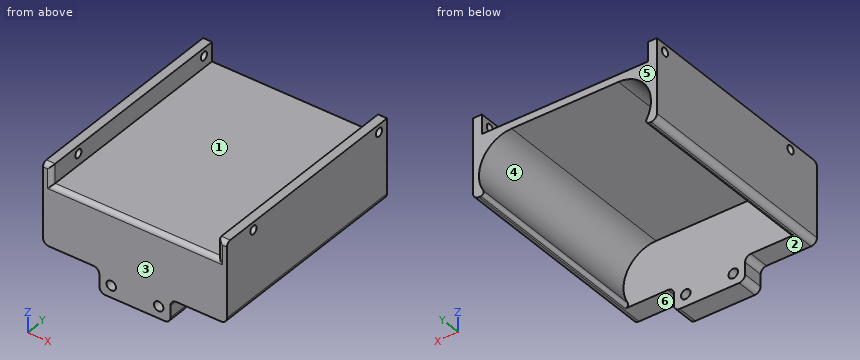
```python
from build123d import *

# Parameters (mm, degrees)
BOSS_EXTRUDE1_DEPTH = 72
CUT_EXTRUDE1_DEPTH  = 65
FILLET3_R           = 2
FILLET4_R           = 1.5
SKETCH5_R           = 1.4
CUT_EXTRUDE2_DEPTH  = 96.970047411
SKETCH6_W           = 24
SKETCH6_H           = 8
BOSS_EXTRUDE3_DEPTH = 7
FILLET5_R           = 2
SKETCH7_R           = 1.6
CUT_EXTRUDE3_DEPTH  = 7
FILLET6_R           = 1


with BuildPart() as part:
    # Sketch1 → Boss-Extrude1 (new body)
    with BuildSketch(Plane(origin=(0, 0, 0), x_dir=(1, 0, 0), z_dir=(0, 1, 0))):
        Polygon((-31, 13.5), (-31, -13.5), (-28, -13.5), (-28, -7), (28, -7), (28, -13.5), (31, -13.5), (31, 13.5), (28, 13.5), (-28, 13.5), align=None)
    extrude(amount=BOSS_EXTRUDE1_DEPTH)

    # Sketch2 → Cut-Extrude1 (cut)
    with BuildSketch(Plane(origin=(0, 72, 0), x_dir=(1, 0, 0), z_dir=(0, 1, 0))):
        with BuildLine():
            Line((17.999983181, 17.5), (-18.000016819, 17.500086496))
            ThreePointArc((-18.000016819, 17.500086496), (-29.000086496, 6.499978376), (-17.999973571, -4.500086496))
            Line((-17.999973571, -4.500086496), (18.000026429, -4.5))
            ThreePointArc((18.000026429, -4.5), (29, 6.500021624), (17.999983181, 17.5))
        make_face()
    extrude(amount=-CUT_EXTRUDE1_DEPTH, mode=Mode.SUBTRACT)

    # Fillet3
    fillet3_edges = [part.edges().sort_by_distance(p)[0] for p in [
        (31, 36, -13.5),
        (-31, 36, -13.5),
    ]]
    fillet(fillet3_edges, radius=FILLET3_R)

    # Fillet4
    fillet4_edges = [part.edges().sort_by_distance(p)[0] for p in [
        (29.5, 0, 13.5),
        (28, 0, 10.25),
        (0, 0, 7),
        (-28, 0, 10.25),
        (-29.5, 0, 13.5),
    ]]
    fillet(fillet4_edges, radius=FILLET4_R)

    # Sketch5 → Cut-Extrude2 (cut, through all)
    with BuildSketch(Plane.ZY.offset(31)):
        with Locations((10.9, 68.4)):
            Circle(SKETCH5_R)
        with Locations((10.9, 11.9)):
            Circle(SKETCH5_R)
    extrude(amount=-CUT_EXTRUDE2_DEPTH, mode=Mode.SUBTRACT)

    # Sketch6 → Boss-Extrude3 (add)
    with BuildSketch(Plane(origin=(0, 0, 0), x_dir=(1, 0, 0), z_dir=(0, 1, 0))):
        with Locations((-5.6065e-05, 17.5)):
            Rectangle(SKETCH6_W, SKETCH6_H)
    extrude(amount=BOSS_EXTRUDE3_DEPTH)

    # Fillet5
    fillet5_edges = [part.edges().sort_by_distance(p)[0] for p in [
        (-12.000056065, 3.5, -21.5),
        (-12.000056065, 3.5, -13.5),
        (11.999943935, 3.5, -13.5),
        (11.999943935, 3.5, -21.5),
    ]]
    fillet(fillet5_edges, radius=FILLET5_R)

    # Sketch7 → Cut-Extrude3 (cut)
    with BuildSketch(Plane(origin=(0, 7, 0), x_dir=(1, 0, 0), z_dir=(0, 1, 0))):
        with Locations(Location((-8.000056065, 17.5, 0), (0, 0, 270))):
            Circle(SKETCH7_R)
        with Locations(Location((7.999943935, 17.5, 0), (0, 0, 270))):
            Circle(SKETCH7_R)
    extrude(amount=-CUT_EXTRUDE3_DEPTH, mode=Mode.SUBTRACT)

    # Fillet6
    fillet6_edges = [part.edges().sort_by_distance(p)[0] for p in [
        (26.485281374, 39.5, -13.5),
        (-26.485393504, 39.5, -13.5),
    ]]
    fillet(fillet6_edges, radius=FILLET6_R)


solid = part.part
```
Model file for the job. Use its own axes, mm. Face numbers are marked on the shaded views. A direction names the side the tool comes from. Round coordinates to 2 decimals unless told otherwise and drop trailing zeros. Write each loop counter-clockwise with the first axis right and the second up, starting at its lowest first coordinate (ties: lowest second). Pieces come first, ordered by that corner, then holes. Notation, with made-up numbers: (-33.75, -18.5) - (-6.75, -18.5) arc R17 ccw to (-6.75, -4.5) - close; hole circle Ø9 at (66, 42.5). An arc over 180 degrees is marked (long way). One line per item, written item: value.
(1) Wall check: probe 1 along X at (y, z) = (2.25, -17.5); probe 2 along Y at (x, z) = (29.9, 10.9); probe 3 along X at (y, z) = (39, -7). Give the ranges that are in metal, low to high.
Values follow:
probe 1: x = -12 to -9.6, -6.4 to 6.4, 9.6 to 12
probe 2: y = 0 to 10.5, 13.3 to 67, 69.8 to 72
probe 3: x = -31 to -28.99, 28.99 to 31
(2) Cut at C-C, the plane y = 68.4. Give the cut face in (x, z), plus the area to 3 significant figures.
Values follow:
outline: (-31, -11.5) arc R2 ccw to (-29, -13.5) - (-28.39, -13.5) arc R1 ccw to (-27.53, -12) arc R11 cw to (-18, 4.5) - (18, 4.5) arc R11 cw to (27.53, -12) arc R1 ccw to (28.39, -13.5) - (29, -13.5) arc R2 ccw to (31, -11.5) - (31, 9.5) - (28, 9.5) - (28, 7) - (-28, 7) - (-28, 9.5) - (-31, 9.5) - close; (-31, 12.3) - (-28, 12.3) - (-28, 13.5) - (-31, 13.5) - close; (28, 12.3) - (31, 12.3) - (31, 13.5) - (28, 13.5) - close
area: 309 mm²
(3) Cut at B-B, the plane z = -17.5. Give the cut face in (x, y).
Values follow:
outline: (-12, 0) - (-9.6, 0) - (-9.6, 7) - (-12, 7) - close; (-6.4, 0) - (6.4, 0) - (6.4, 7) - (-6.4, 7) - close; (9.6, 0) - (12, 0) - (12, 7) - (9.6, 7) - close
(4) Cut at A-A, the plane z = 8. Give the cut face in (x, y), plus the area to 3 significant figures.
Values follow:
outline: (-31, 0) - (-29.5, 0) arc R1.5 ccw to (-28, 1.5) - (-28, 72) - (-31, 72) - close; (28, 1.5) arc R1.5 ccw to (29.5, 0) - (31, 0) - (31, 72) - (28, 72) - close
area: 431 mm²
(5) Drop flat-ended pins along their axis: P1, Ø3, axis at x = 8, z = -17.5, coming from the +Y side; P2, Ø8, axis at x = -14.5, z = -9.5, coming from the +Y side; P3, Ø6, axis at x = -21, z = 9.5, coming from the -Y side; P4, Ø4.5, axis at y = 2, z = -17.5, coming from the -X side. Give the stop position or say it passes through.
Values follow:
P1: passes through
P2: stops at y = 7
P3: stops at y = 0.38
P4: stops at x = -12.02
(6) Two-plate mould, pull along Z, no slides. Class the marked faces 4, 5 and 6: pulls with the +Z half, pulls with the -Z half, needs draft (parallel to the pull), parting line crosses it, or undercut.
Values follow:
face 4: undercut
face 5: needs draft
face 6: pulls with the -Z half
(7) Cut at D-D, the plane x = 19. Give the cut face in (y, z).
Values follow:
outline: (0, -13.5) - (7, -13.5) - (7, 4.45) - (72, 4.45) - (72, 7) - (1.5, 7) arc R1.5 ccw to (0, 5.5) - close
(8) 3-axis set-ups, long thin cutter, end or side, ignore diameter. For the marked faces 1, 2 and 3: which of +Z, -Z, +X, -X, +Y, -Y reach the whole face in a straight line?
Values follow:
face 1: +Z, +Y, -Y
face 2: -Z, -X, +Y, -Y
face 3: +Z, -Z, +X, -X, -Y
